Here's how the part is built. I have some questions about the finished solid (model axes, mm). A direction names the side the tool comes from. Round coordinates to 2 decimals unless told otherwise and drop trailing zeros. Loops run counter-clockwise (first coordinate to the right, second up) from the corner with the lowest first, then second, coordinate; pieces in that order, holes last. Notation, with made-up numbers: M -14,27.25 L 11,27.25 A12 cw 11,39.25 Z; hole C -34.75,-26.5 d2. An arc over 180 degrees is marked long. Answer as a JSON object with one key per item and string values.
from build123d import *

# Parameters (mm, degrees)
SKETCH2_R          = 4
REVOLVE7_ANGLE     = 180
CUT_EXTRUDE1_START = -2
SKETCH6_W          = 1.5
SKETCH6_H          = 8
CUT_EXTRUDE1_DEPTH = 12
SKETCH8_R          = 0.75
CUT_EXTRUDE2_DEPTH = 1.5


with BuildPart() as part:
    # Sweep1: sweep along a path in Sketch1
    with BuildLine(Plane.XY) as sweep1_path:
        Line((-181.381279793, 177.381279793), (-177.381279793, 177.381279793))
        Line((-177.381279793, 177.381279793), (177.381279793, -177.381279793))
        Line((177.381279793, -177.381279793), (177.381279793, -181.381279793))
    # Sketch2 → Sweep1 (sweep)
    with BuildSketch(Plane(origin=(0, 0, 0), x_dir=(0, 0, 1), z_dir=(-0.707106781, 0.707106781, 0))):
        Circle(SKETCH2_R)
    sweep(path=sweep1_path.line, transition=Transition.RIGHT)

    # Sketch4 → Revolve7 (revolve)
    with BuildSketch(Plane.XZ.offset(181.381279793)):
        with BuildLine():
            Line((177.381279793, 4), (177.381279793, -4))
            ThreePointArc((177.381279793, -4), (181.381279793, 0), (177.381279793, 4))
        make_face()
    revolve7 = revolve(axis=Axis((177.381279793, -181.381279793, 4), (0, 0, -1)), revolution_arc=REVOLVE7_ANGLE)

    # Sketch6 → Cut-Extrude1 (cut)
    with BuildSketch(Plane(origin=(0, -181.381279793, 0), x_dir=(-1, 0, 0), z_dir=(0, -1, 0)).offset(CUT_EXTRUDE1_START)):
        with Locations((-177.381279793, 0)):
            Rectangle(SKETCH6_W, SKETCH6_H)
    cut_extrude1 = extrude(amount=CUT_EXTRUDE1_DEPTH, mode=Mode.SUBTRACT)

    # Sketch8 → Cut-Extrude2 (cut, symmetric)
    with BuildSketch(Plane(origin=(177.381279793, 0, 0), x_dir=(0, 0, -1), z_dir=(1, 0, 0))):
        with Locations((0, -182.310338204)):
            Circle(SKETCH8_R)
    cut_extrude2 = extrude(amount=CUT_EXTRUDE2_DEPTH, both=True, mode=Mode.SUBTRACT)

    # Mirror1: Revolve7, Cut-Extrude1, Cut-Extrude2 across plane
    add(revolve7.mirror(Plane(origin=(0, 0, 0), x_dir=(0, 0, 1), z_dir=(-0.707106781, 0.707106781, 0))))
    add(cut_extrude1.mirror(Plane(origin=(0, 0, 0), x_dir=(0, 0, 1), z_dir=(-0.707106781, 0.707106781, 0))), mode=Mode.SUBTRACT)
    add(cut_extrude2.mirror(Plane(origin=(0, 0, 0), x_dir=(0, 0, 1), z_dir=(-0.707106781, 0.707106781, 0))), mode=Mode.SUBTRACT)


solid = part.part
Item 1: I'm going to push flat-ended pins straight in: pin 1 Ø1.4 at (x, z) = (-182.31, 0) entering from +Y; pin 2 Ø1.4 at (y, z) = (-182.31, 0) entering from -X; pin 3 Ø4 at (y, z) = (8, -2.5) entering from -X. Where does each tip first touch, or does it pass through?
Resolved:
{"pin 1": "y = 181.37", "pin 2": "x = 173.39", "pin 3": "x = -14.98"}
Item 2: On a 3-axis mill with a long thin cutter (end or side, diameter ignored), from which of +Z, -Z, +X, -X, +Y, -Y can I reach the whole of each face in a straight line? I mean faces 1 (the face through (-179.14, 180.93, 1.85)), 2 (the face through (5.26, 0.26, -0.87)), 3 (the face through (180.93, -179.22, 1.85)). Say none if no direction works.
Resolved:
{"face 1": "-X", "face 2": "none", "face 3": "-Y"}
Item 3: I want a section at A-A, the plane z = -2. Please give me the cut outline in (x, y), then the cut area to 3 significant figures.
Resolved:
{"outline": "M -184.76,176.63 A3.46 ccw -181.38,173.92 L -178.82,173.92 L 173.92,-178.82 L 173.92,-181.38 A3.46 ccw 176.63,-184.76 L 176.63,-179.38 L 178.13,-179.38 L 178.13,-184.76 A3.46 ccw 180.85,-181.38 L 180.85,-175.95 L -175.95,180.85 L -181.38,180.85 A3.46 ccw -184.76,178.13 L -179.38,178.13 L -179.38,176.63 Z", "area": "3,550 mm²"}
Item 4: Please list where these lines run through material, in increasing order: probe 1 along Y at (x, z) = (139.5, 2.25); probe 2 along Y at (x, z) = (41, -1.5); probe 3 along X at (y, z) = (-68, 1). Write a range as from..to.
Resolved:
{"probe 1": "-144.18..-134.82", "probe 2": "-46.24..-35.76", "probe 3": "62.52..73.48"}
